from build123d import *

# Parameters (mm, degrees)
BOSS_EXTRUDE1_DEPTH = 710
CUT_EXTRUDE2_DEPTH  = 10
SKETCH2_R           = 4.5
CUT_EXTRUDE3_DEPTH  = 10


with BuildPart() as part:
    # Sketch1 → Boss-Extrude1 (new body)
    with BuildSketch(Plane.XY):
        Polygon((-9.451520251, 23.80952381), (-9.451520251, -26.19047619), (15.548479749, -26.19047619), (15.548479749, -23.69047619), (-6.951520251, -23.69047619), (-6.951520251, 23.80952381), align=None)
    extrude(amount=BOSS_EXTRUDE1_DEPTH)

    # Sketch3 → Cut-Extrude2 (cut)
    with BuildSketch(Plane(origin=(0, -23.69047619, 0), x_dir=(1, 0, 0), z_dir=(0, 1, 0))):
        with BuildLine():
            Line((0.571135038, -219.92842441), (0.571135038, -200.92842441))
            ThreePointArc((0.571135038, -200.92842441), (4.071135038, -198.06459908), (7.571135038, -200.92842441))
            Line((7.571135038, -200.92842441), (7.571135038, -219.92842441))
            ThreePointArc((7.571135038, -219.92842441), (4.071135038, -223.510363015), (0.571135038, -219.92842441))
        make_face()
        with BuildLine():
            Line((0.569964611, -115.462655238), (0.570877182, -96.46265526))
            ThreePointArc((0.570877182, -96.46265526), (4.072165698, -92.963944251), (7.570876708, -96.465232767))
            Line((7.570876708, -96.465232767), (7.571895363, -115.465232739))
            ThreePointArc((7.571895363, -115.465232739), (4.069587599, -119.110618262), (0.569964611, -115.462655238))
        make_face()
        with BuildLine():
            Line((0.583868221, -24.003598612), (0.583868221, -6.003598612))
            ThreePointArc((0.583868221, -6.003598612), (4.083868221, -2.503598612), (7.583868221, -6.003598612))
            Line((7.583868221, -6.003598612), (7.583868221, -24.003598612))
            ThreePointArc((7.583868221, -24.003598612), (4.083868221, -27.503598612), (0.583868221, -24.003598612))
        make_face()
        with BuildLine():
            Line((0.551168836, -304.990076897), (0.551168836, -285.990076897))
            ThreePointArc((0.551168836, -285.990076897), (4.051168836, -282.538492606), (7.551168836, -285.990076897))
            Line((7.551168836, -285.990076897), (7.551168836, -304.990076897))
            ThreePointArc((7.551168836, -304.990076897), (4.051168836, -308.572015501), (0.551168836, -304.990076897))
        make_face()
        with BuildLine():
            Line((0.549325866, -377.049780646), (0.549325866, -358.049780646))
            ThreePointArc((0.549325866, -358.049780646), (4.049325866, -354.598196355), (7.549325866, -358.049780646))
            Line((7.549325866, -358.049780646), (7.549325866, -377.049780646))
            ThreePointArc((7.549325866, -377.049780646), (4.049325866, -380.63171925), (0.549325866, -377.049780646))
        make_face()
        with BuildLine():
            Line((0.543910271, -461.67525715), (0.543910271, -442.67525715))
            ThreePointArc((0.543910271, -442.67525715), (4.043910271, -439.223672859), (7.543910271, -442.67525715))
            Line((7.543910271, -442.67525715), (7.543910271, -461.67525715))
            ThreePointArc((7.543910271, -461.67525715), (4.043910271, -465.257195754), (0.543910271, -461.67525715))
        make_face()
        with BuildLine():
            Line((0.482021973, -538.640227915), (0.482021973, -519.640227915))
            ThreePointArc((0.482021973, -519.640227915), (3.982021973, -516.188643625), (7.482021973, -519.640227915))
            Line((7.482021973, -519.640227915), (7.482021973, -538.640227915))
            ThreePointArc((7.482021973, -538.640227915), (3.982021973, -542.22216652), (0.482021973, -538.640227915))
        make_face()
        with BuildLine():
            Line((0.537615818, -621.781220279), (0.537615818, -602.781220279))
            ThreePointArc((0.537615818, -602.781220279), (4.037615818, -599.329635989), (7.537615818, -602.781220279))
            Line((7.537615818, -602.781220279), (7.537615818, -621.781220279))
            ThreePointArc((7.537615818, -621.781220279), (4.037615818, -625.363158884), (0.537615818, -621.781220279))
        make_face()
        with BuildLine():
            Line((0.532196004, -692.166466569), (0.532196004, -673.166466569))
            ThreePointArc((0.532196004, -673.166466569), (4.032196004, -669.714882279), (7.532196004, -673.166466569))
            Line((7.532196004, -673.166466569), (7.532196004, -692.166466569))
            ThreePointArc((7.532196004, -692.166466569), (4.032196004, -695.748405174), (0.532196004, -692.166466569))
        make_face()
    extrude(amount=-CUT_EXTRUDE2_DEPTH, mode=Mode.SUBTRACT)

    # Sketch2 → Cut-Extrude3 (cut)
    with BuildSketch(Plane(origin=(-6.951520251, 0, 0), x_dir=(0, 0, -1), z_dir=(1, 0, 0))):
        with Locations(Location((-649.198051525, 6.719410966, 0), (0, 0, 90))):
            Circle(SKETCH2_R)
        with Locations(Location((-612.198051525, 6.716309021, 0), (0, 0, 90))):
            Circle(SKETCH2_R)
        with Locations(Location((-575.198051525, 6.713207076, 0), (0, 0, 90))):
            Circle(SKETCH2_R)
        with Locations(Location((-242.198051785, 6.685289571, 0), (0, 0, 90))):
            Circle(SKETCH2_R)
        with Locations(Location((-279.198051785, 6.688391516, 0), (0, 0, 90))):
            Circle(SKETCH2_R)
        with Locations(Location((-538.198051525, 6.710105131, 0), (0, 0, 90))):
            Circle(SKETCH2_R)
        with Locations(Location((-501.198051525, 6.707003186, 0), (0, 0, 90))):
            Circle(SKETCH2_R)
        with Locations(Location((-464.198051525, 6.703901241, 0), (0, 0, 90))):
            Circle(SKETCH2_R)
        with Locations(Location((-427.198051525, 6.700799296, 0), (0, 0, 90))):
            Circle(SKETCH2_R)
        with Locations(Location((-390.198051525, 6.697697351, 0), (0, 0, 90))):
            Circle(SKETCH2_R)
        with Locations(Location((-353.198051655, 6.694595406, 0), (0, 0, 90))):
            Circle(SKETCH2_R)
        with Locations(Location((-316.198051785, 6.691493461, 0), (0, 0, 90))):
            Circle(SKETCH2_R)
        with Locations(Location((-686.198051395, 6.722512911, 0), (0, 0, 90))):
            Circle(SKETCH2_R)
        with Locations(Location((-24.198051395, 6.667013246, 0), (0, 0, 90))):
            Circle(SKETCH2_R)
        with Locations(Location((-57.198052435, 6.669779846, 0), (0, 0, 90))):
            Circle(SKETCH2_R)
        with Locations(Location((-205.198051915, 6.682187626, 0), (0, 0, 90))):
            Circle(SKETCH2_R)
        with Locations(Location((-168.198052045, 6.679085681, 0), (0, 0, 90))):
            Circle(SKETCH2_R)
        with Locations(Location((-131.198052175, 6.675983736, 0), (0, 0, 90))):
            Circle(SKETCH2_R)
        with Locations(Location((-94.198052305, 6.672881791, 0), (0, 0, 90))):
            Circle(SKETCH2_R)
    extrude(amount=-CUT_EXTRUDE3_DEPTH, mode=Mode.SUBTRACT)


solid = part.part
Design review of the part built by this model. Coordinates are the model's own, in mm. A direction names the side the tool comes from. Round coordinates to 2 decimals unless told otherwise and drop trailing zeros. Write each loop counter-clockwise with the first axis right and the second up, starting at its lowest first coordinate (ties: lowest second). Pieces come first, ordered by that corner, then holes.
Item 1: Consider section B-B on x = 11.75. Give the boundary of the cut face in (y, z).
Item 2: Wall thickness on L1, parallel to Y at x = -4.75, z = 47; L2, parallel to X at y = 21.5, z = 622.5: over which ranges is each line inside the solid? List them lowest first.
Item 3: For pin 1 Ø11.5 at (y, z) = (6.72, 612.2) entering from +X; pin 2 Ø6 at (x, z) = (0.5, 531) entering from +Y, all flat-tipped, find the tip position at first contact; note any pin that passes through.
Item 4: For faces 1 (the flat face through (-6.952, 0, 350)), 2 (the flat face through (-9.452, -1, 350)), list the 3-axis set-ups (+Z, -Z, +X, -X, +Y, -Y) from which the entire face can be reached by the end or side of a thin tool; tool diameter is ignored.
Item 5: Consider section A-A on y = -15. Give the boundary of the cut face in (x, z), and give its area (4 significant figures).
Check values:
1. outline: (-26.19, 0) - (-23.69, 0) - (-23.69, 710) - (-26.19, 710) - close
2. L1: y = -26.19 to -23.69
2. L2: x = -9.45 to -6.95
3. pin 1: stops at x = -6.95
3. pin 2: stops at y = -23.69
4. face 1: +Z, -Z, +X, +Y
4. face 2: +Z, -Z, -X, +Y, -Y
5. outline: (-9.45, 0) - (-6.95, 0) - (-6.95, 710) - (-9.45, 710) - close
5. area: 1,775 mm2
